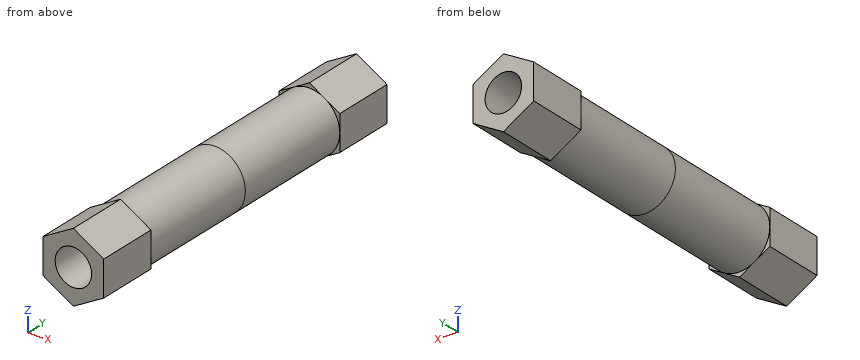
```python
from build123d import *

# Parameters (mm, degrees)
F1_R     = 2.5
F2_DEPTH = 10
F4_DEPTH = 5
F5_D     = 3


# Not quite as in the source:
# - a feature names something its author has since deleted; it is built from what else it names


with BuildPart() as f2:
    # F1 (on Front) → F2 (new body)
    with BuildSketch(Plane.XZ):
        Circle(F1_R)
    extrude(amount=F2_DEPTH)

    # F3 (on face) → F4 (join)
    with BuildSketch(Plane.XZ.offset(10)):
        Polygon((-2.5, 1.443375673), (-2.5, -1.443375673), (0, -2.8867513459), (2.5, -1.443375673), (2.5, 1.443375673), (0, 2.8867513459), align=None)
    extrude(amount=F4_DEPTH)

    # F5 (through all)
    with Locations(Plane(origin=(0, 0, 0), x_dir=(1, 0, 0), z_dir=(0, 1, 0))):
        with Locations((0, 0)):
            Hole(F5_D / 2)

    # F6: F2 across face


with BuildPart() as f2_1:
    add(f2.part)
    add(f2.part.mirror(Plane.XZ))


solid = f2_1.part
```
Geometry check sheet. Reference: the model listing, model coordinates, mm. Coordinates: 2 decimals unless noted, no trailing zeros. Order: outer loops, then holes, each group sorted by start corner. A loop starts at its lowest first (then second) coordinate and runs counter-clockwise, first axis right, second up.
Item 1: Section check B-B (z = 0.7). Enter the section's corners in (x, y), plus the area to 3 significant figures.
Item 2: Section check D-D (x = -1.8). Enter the section's corners in (y, z), plus the area to 3 significant figures.
Item 3: Scan lines: line 1 along Y through (x, z) = (0.1, -2.6); line 2 along Z through (x, y) = (0, -4). Record each from-to range of solid material in increasing order.
Item 4: Depth check by flat-ended pin: pin 1 (3 mm diameter, centred on y = -3.5, z = -2, fed in from -X); pin 2 (1 mm diameter, centred on x = 0, y = -2, fed in from -Z). Enter the tip coordinate at first touch or a pass-through.
Item 5: Section check C-C (x = -0.25). Enter the section's corners in (y, z).
Item 6: Section check A-A (y = 11.25). Enter the section's corners in (x, z).
Check sheet entries:
1. outline: (-2.5, -15) - (-1.33, -15) - (-1.33, 15) - (-2.5, 15) - (-2.5, 10) - (-2.4, 10) - (-2.4, -10) - (-2.5, -10) - close; (1.33, -15) - (2.5, -15) - (2.5, -10) - (2.4, -10) - (2.4, 10) - (2.5, 10) - (2.5, 15) - (1.33, 15) - close
1. area: 66.4 mm2
2. outline: (-15, -1.85) - (-10, -1.85) - (-10, -1.73) - (10, -1.73) - (10, -1.85) - (15, -1.85) - (15, 1.85) - (10, 1.85) - (10, 1.73) - (-10, 1.73) - (-10, 1.85) - (-15, 1.85) - close
2. area: 106 mm2
3. line 1: y = -15 to -10, 10 to 15
3. line 2: z = -2.5 to -1.5, 1.5 to 2.5
4. pin 1: stops at x = -2.45
4. pin 2: stops at z = -2.5
5. outline: (-15, -2.74) - (-10, -2.74) - (-10, -2.49) - (10, -2.49) - (10, -2.74) - (15, -2.74) - (15, -1.48) - (-15, -1.48) - close; (-15, 1.48) - (15, 1.48) - (15, 2.74) - (10, 2.74) - (10, 2.49) - (-10, 2.49) - (-10, 2.74) - (-15, 2.74) - close
6. outline: (-2.5, -1.44) - (0, -2.89) - (2.5, -1.44) - (2.5, 1.44) - (0, 2.89) - (-2.5, 1.44) - close; hole circle Ø3 at (0, 0)
